from build123d import *

# Parameters (mm, degrees)
SKETCH1_R           = 3
SKETCH1_R_2         = 1
BOSS_EXTRUDE1_DEPTH = 3.5
SKETCH2_R           = 2
SKETCH2_R_2         = 1
BOSS_EXTRUDE2_DEPTH = 1.6
SKETCH3_R           = 3
SKETCH3_R_2         = 1
BOSS_EXTRUDE3_DEPTH = 2
FILLET1_R           = 0.25


with BuildPart() as part:
    # Sketch1 → Boss-Extrude1 (new body)
    with BuildSketch(Plane(origin=(0, 0, 0), x_dir=(1, 0, 0), z_dir=(0, 1, 0))):
        Circle(SKETCH1_R)
        Circle(SKETCH1_R_2, mode=Mode.SUBTRACT)
    extrude(amount=BOSS_EXTRUDE1_DEPTH)

    # Sketch2 → Boss-Extrude2 (add)
    with BuildSketch(Plane(origin=(0, 3.5, 0), x_dir=(1, 0, 0), z_dir=(0, 1, 0))):
        Circle(SKETCH2_R)
        Circle(SKETCH2_R_2, mode=Mode.SUBTRACT)
    extrude(amount=BOSS_EXTRUDE2_DEPTH)

    # Sketch3 → Boss-Extrude3 (add)
    with BuildSketch(Plane(origin=(0, 5.1, 0), x_dir=(1, 0, 0), z_dir=(0, 1, 0))):
        Circle(SKETCH3_R)
        Circle(SKETCH3_R_2, mode=Mode.SUBTRACT)
    extrude(amount=BOSS_EXTRUDE3_DEPTH)

    # Fillet1
    fillet1_edges = [part.edges().sort_by_distance(p)[0] for p in [
        (-3, 7.1, 0),
        (-3, 0, 0),
    ]]
    fillet(fillet1_edges, radius=FILLET1_R)


solid = part.part
The model under review builds one solid part; all positions refer to its coordinate system, in mm. A direction names the side the tool comes from. Coordinates: 2 decimals unless noted, no trailing zeros. Loops run counter-clockwise (first coordinate to the right, second up) from the corner with the lowest first, then second, coordinate; pieces in that order, holes last.
(1) Consider section B-B, the plane z = 0. Give the boundary of the cut face in (x, y), plus the area to 3 significant figures.
Determined:
outline: (-3, 0.25) arc R0.25 ccw to (-2.75, 0) - (-1, 0) - (-1, 7.1) - (-2.75, 7.1) arc R0.25 ccw to (-3, 6.85) - (-3, 5.1) - (-2, 5.1) - (-2, 3.5) - (-3, 3.5) - close; (1, 0) - (2.75, 0) arc R0.25 ccw to (3, 0.25) - (3, 3.5) - (2, 3.5) - (2, 5.1) - (3, 5.1) - (3, 6.85) arc R0.25 ccw to (2.75, 7.1) - (1, 7.1) - close
area: 25.1 mm2
(2) Consider section D-D, the plane y = 1.5. Give the boundary of the cut face in (x, z).
Determined:
outline: circle Ø6 at (0, 0); hole circle Ø2 at (0, 0)
(3) Draft analysis for pull direction Y (two halves, no side actions). For faces 1 (the flat face through (1, 3.5, 2)), 2 (the flat face through (0, 0, 1.2)), 3 (the flat face through (0, 7.1, 1.2)), state which applies: +Y half, -Y half, draft (parallel to the pull), parting line (faces both ways), or undercut.
Determined:
face 1: undercut
face 2: -Y half
face 3: +Y half
(4) Consider section C-C, the plane y = 4.75. Give the boundary of the cut face in (x, z), plus the area to 3 significant figures.
Determined:
outline: circle Ø4 at (0, 0); hole circle Ø2 at (0, 0)
area: 9.42 mm2
(5) Insertion check: P1, Ø1.8, axis at x = 0, z = 0, coming from the -Y side. The pin has a flat end and moves straight along its axis. Give the tip position at first contact, or say it passes through.
Determined:
P1: passes through
(6) Consider section A-A, the plane x = 0. Give the boundary of the cut face in (y, z).
Determined:
outline: (0, -2.75) arc R0.25 ccw to (0.25, -3) - (3.5, -3) - (3.5, -2) - (5.1, -2) - (5.1, -3) - (6.85, -3) arc R0.25 ccw to (7.1, -2.75) - (7.1, -1) - (0, -1) - close; (0, 1) - (7.1, 1) - (7.1, 2.75) arc R0.25 ccw to (6.85, 3) - (5.1, 3) - (5.1, 2) - (3.5, 2) - (3.5, 3) - (0.25, 3) arc R0.25 ccw to (0, 2.75) - close
(7) Wall thickness on L1, parallel to X at y = 2, z = 0; L2, parallel to Y at x = 0, z = 2.75; L3, parallel to Z at x = 0, y = 5: over which ranges is each line inside the solid? List them lowest first.
Determined:
L1: x = -3 to -1, 1 to 3
L2: y = 0 to 3.5, 5.1 to 7.1
L3: z = -2 to -1, 1 to 2
(8) Tool access review of faces 4 (the flat face through (1, 5.1, 2)), 5 (the cylindrical face through (-3, 2, 0)): name each direction out of +Z, -Z, +X, -X, +Y, -Y from which nothing blocks a thin tool from reaching the whole face with its end or side.
Determined:
face 4: none
face 5: +Y, -Y
